from build123d import *

# Parameters (mm, degrees)
SKETCH1_W           = 100
SKETCH1_H           = 100
BOSS_EXTRUDE1_DEPTH = 5
SKETCH2_W           = 5
SKETCH2_H           = 40
BOSS_EXTRUDE2_DEPTH = 8
SKETCH4_R           = 2
CUT_EXTRUDE1_DEPTH  = 8


with BuildPart() as part:
    # Sketch1 → Boss-Extrude1 (new body)
    with BuildSketch(Plane(origin=(0, 0, 0), x_dir=(1, 0, 0), z_dir=(0, 1, 0))):
        Rectangle(SKETCH1_W, SKETCH1_H)
    extrude(amount=BOSS_EXTRUDE1_DEPTH)

    # Sketch2 → Boss-Extrude2 (add)
    with BuildSketch(Plane(origin=(0, 5, 0), x_dir=(1, 0, 0), z_dir=(0, 1, 0))):
        with Locations((21.825, 0)):
            Rectangle(SKETCH2_W, SKETCH2_H)
        with Locations((-34.625, 0)):
            Rectangle(SKETCH2_W, SKETCH2_H)
        with Locations((-21.825, 0)):
            Rectangle(SKETCH2_W, SKETCH2_H)
        with Locations((34.625, 0)):
            Rectangle(SKETCH2_W, SKETCH2_H)
    extrude(amount=BOSS_EXTRUDE2_DEPTH)

    # Sketch4 → Cut-Extrude1 (cut)
    with BuildSketch(Plane(origin=(0, 5, 0), x_dir=(1, 0, 0), z_dir=(0, 1, 0))):
        with Locations(Location((40.2, 36.5, 0), (0, 0, 270))):
            Circle(SKETCH4_R)
        with Locations(Location((40.2, -36.5, 0), (0, 0, 270))):
            Circle(SKETCH4_R)
        with Locations(Location((-40.2, -36.5, 0), (0, 0, 270))):
            Circle(SKETCH4_R)
        with Locations(Location((-40.2, 36.5, 0), (0, 0, 270))):
            Circle(SKETCH4_R)
    extrude(amount=-CUT_EXTRUDE1_DEPTH, mode=Mode.SUBTRACT)


solid = part.part
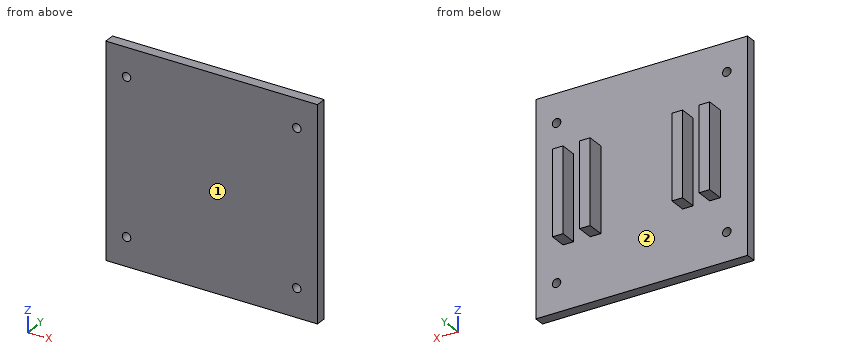
Verification items for the finished model (mm, model axes). Face numbers are marked on the shaded views. Coordinates: 2 decimals unless noted, no trailing zeros. Write each loop counter-clockwise with the first axis right and the second up, starting at its lowest first coordinate (ties: lowest second). Pieces come first, ordered by that corner, then holes. Notation, with made-up numbers: (-10, 55.25) - (1, 55.25) arc R21 ccw to (1, 64.25) - close; hole circle Ø5 at (0.25, 28.5). An arc over 180 degrees is marked (long way). Answer as a JSON object with one key per item and string values.
(1) Gauge pin test, flat ends, axial feed: pin 1 Ø5.5 at (x, y) = (-35.5, 9) entering from +Z; pin 2 Ø2.5 at (y, z) = (7.5, -4.5) entering from +X (3 decimals); pin 3 Ø10 at (x, z) = (-33.5, 6.5) entering from -Y; pin 4 Ø4 at (y, z) = (10.5, 8.5) entering from -X (3 decimals). Record the tip position at first contact, or that the pin passes through.
Report:
{"pin 1": "z = 20", "pin 2": "x = 37.125", "pin 3": "y = 0", "pin 4": "x = -37.125"}
(2) Mould release check, pull along X, two halves, no side actions. Record for the marked faces 1 and 2: pulls with the +X half, pulls with the -X half, needs draft (parallel to the pull), parting line crosses it, or undercut.
Report:
{"face 1": "needs draft", "face 2": "undercut"}
(3) Cross-section at B-B on y = 8.75. Record the cut outline in (x, z) (3 decimals), plus the area to 3 significant figures.
Report:
{"outline": "(-37.125, -20) - (-32.125, -20) - (-32.125, 20) - (-37.125, 20) - close; (-24.325, -20) - (-19.325, -20) - (-19.325, 20) - (-24.325, 20) - close; (19.325, -20) - (24.325, -20) - (24.325, 20) - (19.325, 20) - close; (32.125, -20) - (37.125, -20) - (37.125, 20) - (32.125, 20) - close", "area": "800 mm^2"}
(4) Thickness scan on line 1 along X through (y, z) = (7.5, -2) (3 decimals); line 2 along X through (y, z) = (1.35, -36.5); line 3 along Z through (x, y) = (-39.5, 1). Record the ranges inside material, lowest first.
Report:
{"line 1": "-37.125 to -32.125, -24.325 to -19.325, 19.325 to 24.325, 32.125 to 37.125", "line 2": "-50 to -42.2, -38.2 to 38.2, 42.2 to 50", "line 3": "-50 to -38.37, -34.63 to 34.63, 38.37 to 50"}
(5) Cross-section at D-D on z = 9. Record the cut outline in (x, y) (3 decimals), plus the area to 3 significant figures.
Report:
{"outline": "(-50, 0) - (50, 0) - (50, 5) - (37.125, 5) - (37.125, 13) - (32.125, 13) - (32.125, 5) - (24.325, 5) - (24.325, 13) - (19.325, 13) - (19.325, 5) - (-19.325, 5) - (-19.325, 13) - (-24.325, 13) - (-24.325, 5) - (-32.125, 5) - (-32.125, 13) - (-37.125, 13) - (-37.125, 5) - (-50, 5) - close", "area": "660 mm^2"}
(6) Cross-section at C-C on z = 36.5. Record the cut outline in (x, y).
Report:
{"outline": "(-50, 0) - (-42.2, 0) - (-42.2, 5) - (-50, 5) - close; (-38.2, 0) - (38.2, 0) - (38.2, 5) - (-38.2, 5) - close; (42.2, 0) - (50, 0) - (50, 5) - (42.2, 5) - close"}
(7) Cross-section at A-A on x = 40.2. Record the cut outline in (y, z), plus the area to 3 significant figures.
Report:
{"outline": "(0, -50) - (5, -50) - (5, -38.5) - (0, -38.5) - close; (0, -34.5) - (5, -34.5) - (5, 34.5) - (0, 34.5) - close; (0, 38.5) - (5, 38.5) - (5, 50) - (0, 50) - close", "area": "460 mm^2"}
